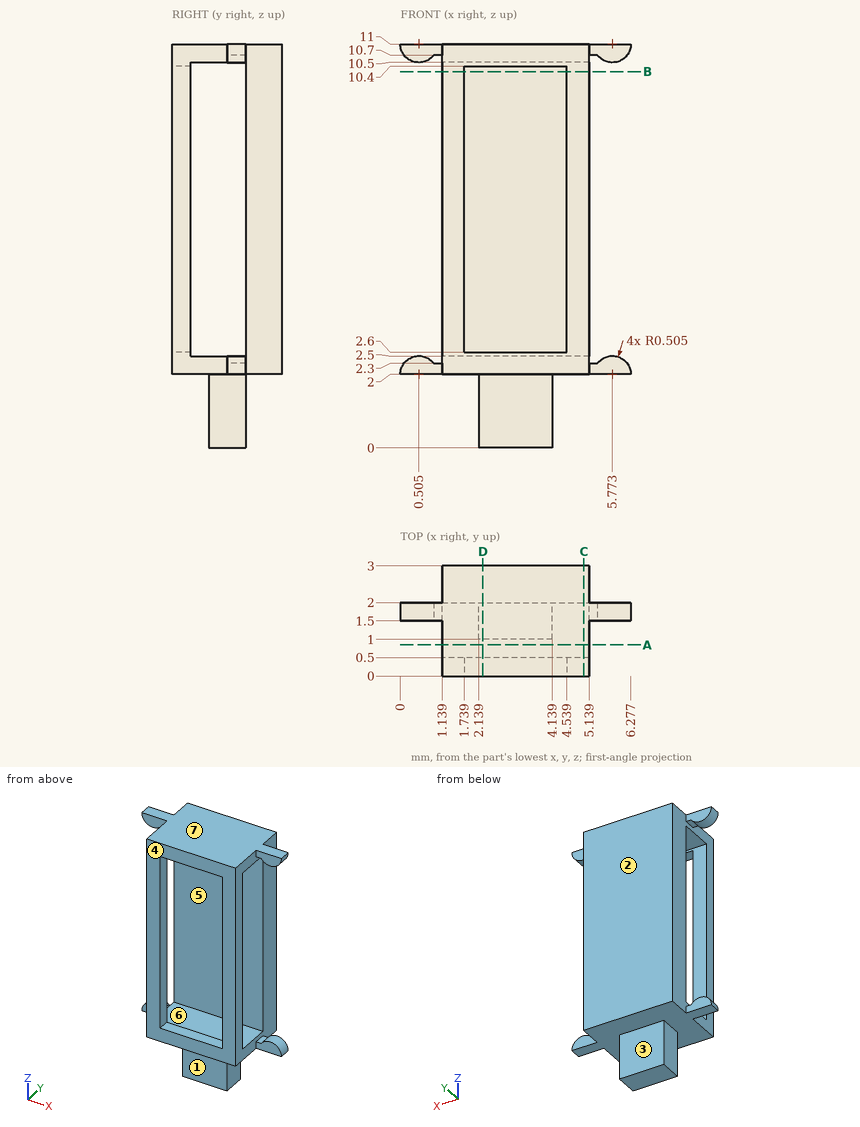
Answer from the drawing. Dimensions are ordinates in mm from the lowest x, y and z of the part. A direction names the side the tool comes from. Coordinates: 2 decimals unless noted, no trailing zeros. Loops run counter-clockwise (first coordinate to the right, second up) from the corner with the lowest first, then second, coordinate; pieces in that order, holes last. Notation, with made-up numbers: (67, 51) - (73, 51) arc R26 cw to (73, 70) - close; hole circle Ø4 at (-40, 63). An arc over 180 degrees is marked (long way). Use a Markdown table: item, result.
Item 1: Find section C-C, the plane x = 5. Determine the outline of the cut face in (y, z), and give its area (3 significant figures).
Evaluation:
| item | result |
|---|---|
| outline | (0, 2) - (3, 2) - (3, 11) - (0, 11) - close; hole (0.5, 2.5) - (2, 2.5) - (2, 10.5) - (0.5, 10.5) - close |
| area | 15.0 mm2 |
Item 2: Given pin 1 Ø0.6 at (x, z) = (0.5, 2) entering from -Y; pin 2 Ø0.6 at (x, z) = (0.5, 10.5) entering from +Y; pin 3 Ø1.2 at (x, y) = (4, 1.5) entering from -Z; pin 4 Ø1.5 at (y, z) = (2, 7) entering from +X, each flat-ended and moving along its own axis, determine where each tip first touches the part or whether it passes through.
Evaluation:
| item | result |
|---|---|
| pin 1 | stops at y = 1.5 |
| pin 2 | stops at y = 2 |
| pin 3 | stops at z = 0 |
| pin 4 | stops at x = 5.14 |
Item 3: Find section A-A, the plane y = 0.85. Determine the outline of the cut face in (x, z).
Evaluation:
| item | result |
|---|---|
| outline | (1.14, 2) - (5.14, 2) - (5.14, 2.5) - (1.14, 2.5) - close; (1.14, 10.5) - (5.14, 10.5) - (5.14, 11) - (1.14, 11) - close |
Item 4: Find section D-D, the plane x = 2.25. Determine the outline of the cut face in (y, z).
Evaluation:
| item | result |
|---|---|
| outline | (0, 2) - (1, 2) - (1, 0) - (2, 0) - (2, 2) - (3, 2) - (3, 11) - (0, 11) - (0, 10.4) - (0.5, 10.4) - (0.5, 10.5) - (2, 10.5) - (2, 2.5) - (0.5, 2.5) - (0.5, 2.6) - (0, 2.6) - close |
Item 5: Find section B-B, the plane z = 10.25. Determine the outline of the cut face in (x, y).
Evaluation:
| item | result |
|---|---|
| outline | (1.14, 0) - (1.74, 0) - (1.74, 0.5) - (1.14, 0.5) - close; (1.14, 2) - (5.14, 2) - (5.14, 3) - (1.14, 3) - close; (4.54, 0) - (5.14, 0) - (5.14, 0.5) - (4.54, 0.5) - close |
Item 6: The mould has two halves that part along Z. Classify the marked faces 4, 5, 6 and 7: +Z half, -Z half, draft (parallel to the pull), parting line (faces both ways), or undercut.
Evaluation:
| item | result |
|---|---|
| face 4 | draft |
| face 5 | undercut |
| face 6 | undercut |
| face 7 | +Z half |
Item 7: Consider probe 1 along X at (y, z) = (0.4, 5.5); probe 2 along Y at (x, z) = (3.5, 9.5); probe 3 along Z at (x, y) = (3, 2.05). Determine where each line is inside the solid, lowest interval first. Write a range as from..to.
Evaluation:
| item | result |
|---|---|
| probe 1 | x = 1.14..1.74, 4.54..5.14 |
| probe 2 | y = 2..3 |
| probe 3 | z = 2..11 |
Item 8: For the marked faces 1, 2 and 3, determine the directions among +Z, -Z, +X, -X, +Y, -Y from which every point of the face is accessible in a straight line to the end or side of a thin tool.
Evaluation:
| item | result |
|---|---|
| face 1 | -Z, +X, -X, -Y |
| face 2 | +Z, -Z, +X, -X, +Y |
| face 3 | -Z, +X, -X, +Y |
